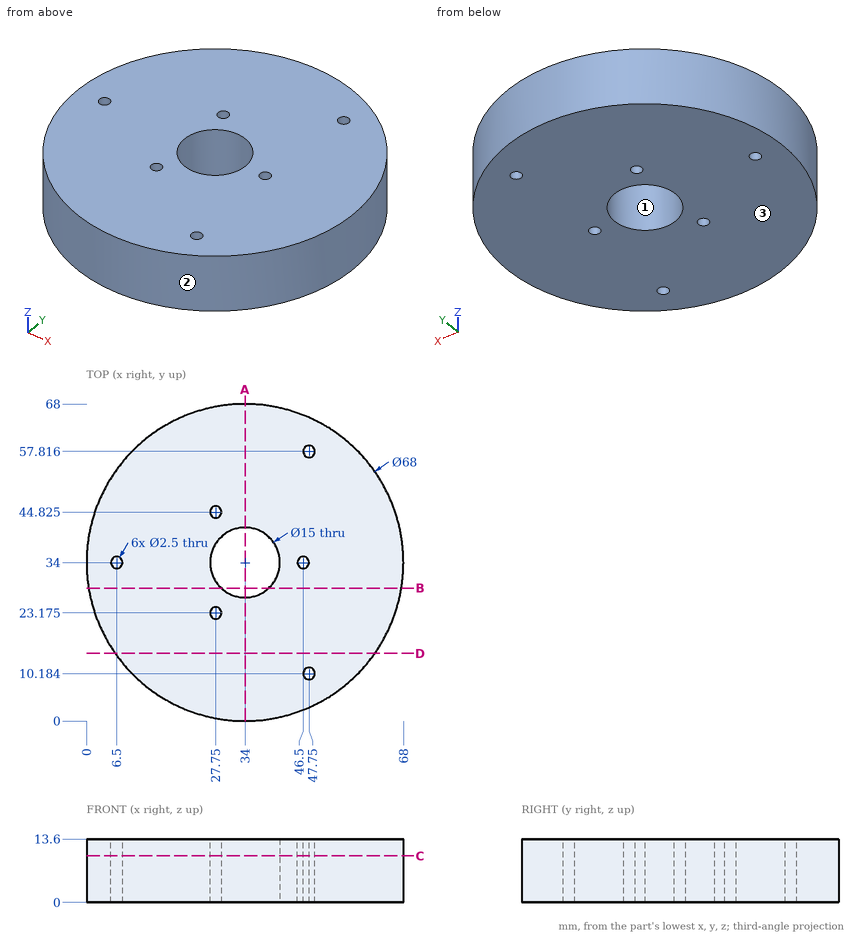
Geometry: see drawing. Coordinates: mm, zero at the bounding-box minimum. Round coordinates to 2 decimals unless told otherwise and drop trailing zeros. Loops run counter-clockwise (first coordinate to the right, second up) from the corner with the lowest first, then second, coordinate; pieces in that order, holes last. Notation, with made-up numbers: (-19, 78.5) -> (5, 78.5) arc R29 ccw to (5, 101.5) -> close; hole circle Ø9 at (70, 25). An arc over 180 degrees is marked (long way). One line per question, with ' | ' between items. Start each with the question number.
1. Line query: line 1 along Y through (x, z) = (28.5, 9.5) (1 decimal); line 2 along Y through (x, z) = (32, 1.5); line 3 along X through (y, z) = (58, 8.5) (1 decimal). Output: solid intervals per line, ascending. Write a range as [from, to].
2. Section C-C on z = 10. Count the separate pieces of the cut face and the enclosed holes in it, and give its area (3 significant figures).
3. Section B-B on y = 28.5. Output: boundary loops of the cut face in (x, z), and give its area (3 significant figures).
4. Mould query, pull axis X, two halves, no side actions, for the marked faces 1, 2 and 3. Classes: pulls with the +X half, pulls with the -X half, needs draft (parallel to the pull), parting line crosses it, or undercut.
5. Section A-A on x = 34. Output: boundary loops of the cut face in (y, z).
6. Section D-D on y = 14.5. Output: boundary loops of the cut face in (x, z).
7. Contact query for flat-ended pins moving along their axis: pin 1 (8 mm diameter, centred on x = 32, z = 12, fed in from +Y); pin 2 (6 mm diameter, centred on y = 16, z = 2, fed in from -X); pin 3 (1.5 mm diameter, centred on y = 14.5, z = 10, fed in from +X). Output: stop coordinate, or through.
Returned:
1) line 1: y = [0.4, 22.2], [24.2, 28.9], [39.1, 43.8], [45.8, 67.6] | line 2: y = [0.06, 26.77], [41.23, 67.94] | line 3: x = [9.9, 46.5], [49, 58.1]
2) separate pieces: 1 | enclosed holes: 7 | area: 3,430 mm2
3) outline: (0.45, 0) -> (28.9, 0) -> (28.9, 13.6) -> (0.45, 13.6) -> close; (39.1, 0) -> (67.55, 0) -> (67.55, 13.6) -> (39.1, 13.6) -> close | area: 774 mm2
4) face 1: undercut | face 2: parting line crosses it | face 3: needs draft
5) outline: (0, 0) -> (26.5, 0) -> (26.5, 13.6) -> (0, 13.6) -> close; (41.5, 0) -> (68, 0) -> (68, 13.6) -> (41.5, 13.6) -> close
6) outline: (6.15, 0) -> (61.85, 0) -> (61.85, 13.6) -> (6.15, 13.6) -> close
7) pin 1: stops at y = 68 | pin 2: stops at x = 3.49 | pin 3: stops at x = 62.36
